Source: CAD feature listing. Evaluate the final solid. Frame: model axes, mm. Face numbers are marked on the shaded views. A direction names the side the tool comes from. Coordinates: 2 decimals unless noted, no trailing zeros. Loops run counter-clockwise (first coordinate to the right, second up) from the corner with the lowest first, then second, coordinate; pieces in that order, holes last. Notation, with made-up numbers: (1, 0) -> (36, 0) arc R25 cw to (36, 19) -> close; hole circle Ø1 at (43.5, 13). An arc over 180 degrees is marked (long way). Answer as CSV lines item,"result".
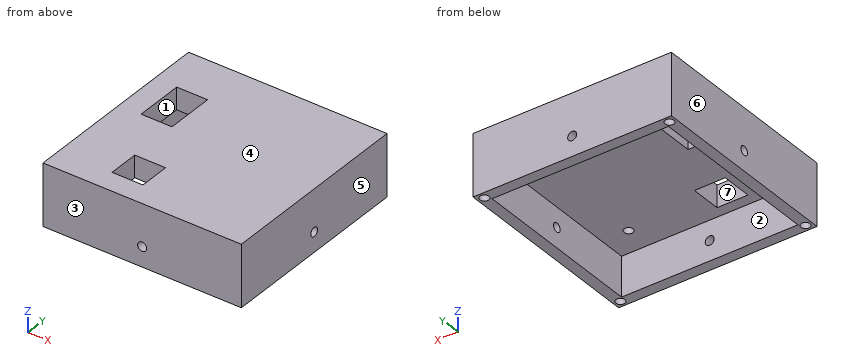
Solid Edge part; units mm, degrees
sketch "Sketch1" plane through (0, 0, 0) normal (0, 0, 1) x (1, 0, 0)
  line L0 (-22.5, -22.5) -> (22.5, -22.5)
  line L1 (22.5, -22.5) -> (22.5, 22.5)
  line L2 (22.5, 22.5) -> (-22.5, 22.5)
  line L3 (-22.5, 22.5) -> (-22.5, -22.5)
  line L4 (-20, -20) -> (20, -20)
  line L5 (20, -20) -> (20, 20)
  line L6 (20, 20) -> (-20, 20)
  line L7 (-20, 20) -> (-20, -20)
extrude "Protrusion1" add sketch "Sketch1" against normal blind 12
sketch "Sketch2" plane through (0, 0, 0) normal (0, 0, 1) x (1, 0, 0)
  line L0 (-20, 20) -> (-20, -20)
  line L1 (-20, -20) -> (20, -20)
  line L2 (20, -20) -> (20, 20)
  line L3 (20, 20) -> (-20, 20)
extrude "ExtrudedProtrusion_2" add sketch "Sketch2" against normal blind 3
sketch "Sketch3" plane through (0, 0, -12) normal (0, 0, -1) x (0, -1, 0)
  circle A0 centre (-21, 21) radius 1.025
  circle A1 centre (-21, -21) radius 1.025
  circle A2 centre (21, -21) radius 1.025
  circle A3 centre (21, 21) radius 1.025
extrude "ExtrudedCutout_1" cut sketch "Sketch3" against normal blind 3.5
sketch "Sketch4" plane through (0, 0, 0) normal (0, 0, 1) x (0, 1, 0)
  line L0 (-17.5, 10.5) -> (-10.5, 10.5)
  line L1 (-10.5, 10.5) -> (-10.5, 3.5)
  line L2 (-10.5, 3.5) -> (-17.5, 3.5)
  line L3 (-17.5, 3.5) -> (-17.5, 10.5)
  line L4 (1, 17.5) -> (12, 17.5)
  line L5 (12, 17.5) -> (12, 10.5)
  line L6 (12, 10.5) -> (1, 10.5)
  line L7 (1, 10.5) -> (1, 17.5)
extrude "Cutout1" cut sketch "Sketch4" along normal through all and the other way through all
sketch "Sketch5" plane through (0, 0, 0) normal (0, 0, 1) x (1, 0, 0)
  line L0 (-22.5, 22.5) -> (-22.5, -22.5)
  line L1 (-22.5, -22.5) -> (22.5, -22.5)
  line L2 (22.5, -22.5) -> (22.5, 22.5)
  line L3 (22.5, 22.5) -> (-22.5, 22.5)
extrude "ExtrudedProtrusion_3" add sketch "Sketch5" along normal blind 2
sketch "Sketch6" plane through (0, 0, 0) normal (0, 0, 1) x (0, 1, 0)
  line L0 (1, 10.5) -> (1, 17.5)
  line L1 (1, 17.5) -> (12, 17.5)
  line L2 (12, 17.5) -> (12, 10.5)
  line L3 (12, 10.5) -> (1, 10.5)
  line L4 (-10.5, 10.5) -> (-10.5, 3.5)
  line L5 (-10.5, 3.5) -> (-17.5, 3.5)
  line L6 (-17.5, 3.5) -> (-17.5, 10.5)
  line L7 (-17.5, 10.5) -> (-10.5, 10.5)
extrude "ExtrudedCutout_4" cut sketch "Sketch6" along normal blind 33.1838
sketch "Sketch7" plane through (0, 0, -3) normal (0, 0, -1) x (0, -1, 0)
  circle A0 centre (-14, 14) radius 1.025
  circle A1 centre (14, 14) radius 1.025
  circle A2 centre (-14, -14) radius 1.025
  circle A3 centre (14, -14) radius 1.025
extrude "ExtrudedCutout_5" cut sketch "Sketch7" against normal blind 3.5
hole "Hole_2" at (20, 0, -7.5) direction (-1, 0, 0) diameter 2.05 end through all both ways yes
hole "Hole_3" at (0, -20, -7.5) direction (0, 1, 0) diameter 2.05 end through all both ways yes
properties part number "BumbleB0361"
(1) Draft query along X for the marked faces 4, 5, 6 and 7. Return one class per face: released by +X, released by -X, zero draft, split by the parting line, or undercut.
Computed values:
face 4,"zero draft"
face 5,"released by +X"
face 6,"released by -X"
face 7,"undercut"
(2) Access query for the marked faces 1, 2 and 3. Directions: +Z, -Z, +X, -X, +Y, -Y. A direction counts if a zero-diameter tool reaches every point of the face in a straight line with its end or side. Return the directions, or none.
Computed values:
face 1,"+Z, -Z"
face 2,"-Z"
face 3,"+Z, -Z, +X, -X, -Y"
(3) Cut plane B-B (x = -21). Return the cut outline in (y, z) (3 decimals).
Computed values:
outline,"(-22.5, -12) -> (-22.025, -12) -> (-22.025, -8.5) -> (-19.975, -8.5) -> (-19.975, -12) -> (19.975, -12) -> (19.975, -8.5) -> (22.025, -8.5) -> (22.025, -12) -> (22.5, -12) -> (22.5, 2) -> (-22.5, 2) -> close; hole circle Ø2.05 at (0, -7.5)"
(4) Cut plane A-A (y = 6). Return the cut outline in (x, z).
Computed values:
outline,"(-22.5, -12) -> (-20, -12) -> (-20, -3) -> (-17.5, -3) -> (-17.5, 2) -> (-22.5, 2) -> close; (-10.5, -3) -> (20, -3) -> (20, -12) -> (22.5, -12) -> (22.5, 2) -> (-10.5, 2) -> close"
(5) Cut plane C-C (z = -7.5). Return the cut outline in (x, y) (3 decimals), then the cut area to 4 significant figures.
Computed values:
outline,"(-22.5, -22.5) -> (-1.025, -22.5) -> (-1.025, -20) -> (-20, -20) -> (-20, -1.025) -> (-22.5, -1.025) -> close; (-22.5, 1.025) -> (-20, 1.025) -> (-20, 20) -> (-1.025, 20) -> (-1.025, 22.5) -> (-22.5, 22.5) -> close; (1.025, -22.5) -> (22.5, -22.5) -> (22.5, -1.025) -> (20, -1.025) -> (20, -20) -> (1.025, -20) -> close; (1.025, 20) -> (20, 20) -> (20, 1.025) -> (22.5, 1.025) -> (22.5, 22.5) -> (1.025, 22.5) -> close"
area,"404.5 mm^2"
(6) Cut plane D-D (x = -14). Return the cut outline in (y, z) (3 decimals), then the cut area to 3 significant figures.
Computed values:
outline,"(-22.5, -12) -> (-20, -12) -> (-20, -3) -> (-15.025, -3) -> (-15.025, 0.5) -> (-12.975, 0.5) -> (-12.975, -3) -> (1, -3) -> (1, 2) -> (-22.5, 2) -> close; (12, -3) -> (12.975, -3) -> (12.975, 0.5) -> (15.025, 0.5) -> (15.025, -3) -> (20, -3) -> (20, -12) -> (22.5, -12) -> (22.5, 2) -> (12, 2) -> close"
area,"201 mm^2"
(7) Material intervals for L1, parallel to X at y = 21, z = -11.2 (3 decimals); L2, parallel to Y at x = 14, z = -2 (3 decimals), sorted ascending. Write a range as [from, to].
Computed values:
L1,"[-22.5, -22.025], [-19.975, 19.975], [22.025, 22.5]"
L2,"[-22.5, -15.025], [-12.975, 12.975], [15.025, 22.5]"
(8) Pin query (flat end, axial travel): pin 1 Ø4 at (x, y) = (7.5, 5.5) entering from -Z; pin 2 Ø3.5 at (x, z) = (0, -7.5) entering from +Y; pin 3 Ø1.6 at (x, y) = (14, 14) entering from -Z. Return the tip coordinate at first contact, or that it passes through.
Computed values:
pin 1,"z = -3"
pin 2,"y = 22.5"
pin 3,"z = 0.5"
